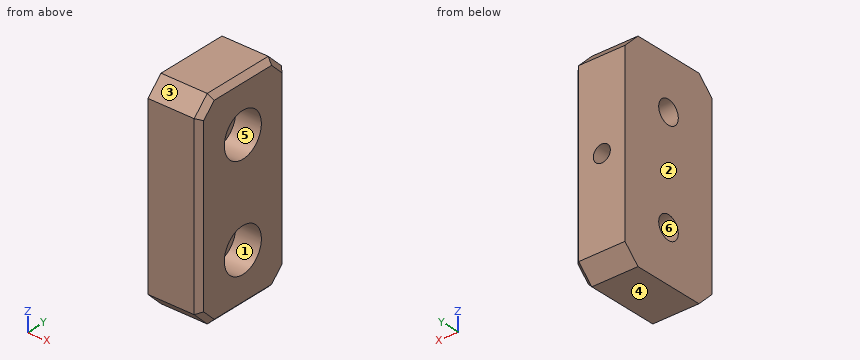
from build123d import *

# Parameters (mm, degrees)
SKETCH1_W           = 40
SKETCH1_H           = 20
BOSS_EXTRUDE1_DEPTH = 10
CHAMFER1_SIZE       = 3
CHAMFER2_SIZE       = 1
CUT_EXTRUDE1_DEPTH  = 10
CUT_EXTRUDE2_DEPTH  = 5
SKETCH3_R           = 1.65
CUT_EXTRUDE3_DEPTH  = 5


with BuildPart() as part:
    # Sketch1 → Boss-Extrude1 (new body)
    with BuildSketch(Plane(origin=(0, 0, 0), x_dir=(0, 0, -1), z_dir=(1, 0, 0))):
        Rectangle(SKETCH1_W, SKETCH1_H)
    extrude(amount=BOSS_EXTRUDE1_DEPTH)

    # Chamfer1
    chamfer1_edges = [part.edges().sort_by_distance(p)[0] for p in [
        (5, -10, -20),
        (5, -10, 20),
        (5, 10, 20),
        (5, 10, -20),
    ]]
    chamfer(chamfer1_edges, length=CHAMFER1_SIZE)

    # Chamfer2
    chamfer2_edges = [part.edges().sort_by_distance(p)[0] for p in [
        (10, 10, 0),
        (10, 0, -20),
        (10, 0, 20),
        (10, -10, 0),
        (10, 8.5, 18.5),
        (10, -8.5, 18.5),
        (10, -8.5, -18.5),
        (10, 8.5, -18.5),
    ]]
    chamfer(chamfer2_edges, length=CHAMFER2_SIZE)

    # Sketch2 → Cut-Extrude1 (cut)
    with BuildSketch(Plane(origin=(10, 0, 0), x_dir=(0, 0, -1), z_dir=(1, 0, 0))):
        with BuildLine():
            ThreePointArc((-12.25, 0), (-10, -2.25), (-7.75, 0))
            Line((-7.75, 0), (-12.25, 0))
        make_face()
        with BuildLine():
            Line((-12.25, 0), (-7.75, 0))
            ThreePointArc((-7.75, 0), (-10, 2.25), (-12.25, 0))
        make_face()
        with BuildLine():
            ThreePointArc((12.25, 0), (10, 2.25), (7.75, 0))
            Line((7.75, 0), (12.25, 0))
        make_face()
        with BuildLine():
            Line((12.25, 0), (7.75, 0))
            ThreePointArc((7.75, 0), (10, -2.25), (12.25, 0))
        make_face()
    extrude(amount=-CUT_EXTRUDE1_DEPTH, mode=Mode.SUBTRACT)

    # Sketch2_3 → Cut-Extrude2 (cut)
    with BuildSketch(Plane(origin=(10, 0, 0), x_dir=(0, 0, -1), z_dir=(1, 0, 0))):
        with BuildLine():
            ThreePointArc((-12.25, 0), (-10, 2.25), (-7.75, 0))
            Line((-7.75, 0), (-5.75, 0))
            ThreePointArc((-5.75, 0), (-10, 4.25), (-14.25, 0))
            Line((-14.25, 0), (-12.25, 0))
        make_face()
        with BuildLine():
            Line((-5.75, 0), (-7.75, 0))
            ThreePointArc((-7.75, 0), (-10, -2.25), (-12.25, 0))
            Line((-12.25, 0), (-14.25, 0))
            ThreePointArc((-14.25, 0), (-10, -4.25), (-5.75, 0))
        make_face()
        with BuildLine():
            ThreePointArc((14.25, 0), (10, 4.25), (5.75, 0))
            Line((5.75, 0), (7.75, 0))
            ThreePointArc((7.75, 0), (10, 2.25), (12.25, 0))
            Line((12.25, 0), (14.25, 0))
        make_face()
        with BuildLine():
            Line((7.75, 0), (5.75, 0))
            ThreePointArc((5.75, 0), (10, -4.25), (14.25, 0))
            Line((14.25, 0), (12.25, 0))
            ThreePointArc((12.25, 0), (10, -2.25), (7.75, 0))
        make_face()
    extrude(amount=-CUT_EXTRUDE2_DEPTH, mode=Mode.SUBTRACT)

    # Sketch3 → Cut-Extrude3 (cut)
    with BuildSketch(Plane(origin=(0, 10, 0), x_dir=(1, 0, 0), z_dir=(0, 1, 0))):
        with Locations((4.5, 0)):
            Circle(SKETCH3_R)
    extrude(amount=-CUT_EXTRUDE3_DEPTH, mode=Mode.SUBTRACT)


solid = part.part
The listing builds one solid part. Answer for the finished solid, in the listing's coordinates (mm). Face numbers are marked on the shaded views. A direction names the side the tool comes from. Give positions to 0.01 mm unless a question says otherwise; leave off trailing zeros. Loops run counter-clockwise (first coordinate to the right, second up) from the corner with the lowest first, then second, coordinate; pieces in that order, holes last. Notation, with made-up numbers: (-27, 44) - (30, 44) arc R10 ccw to (30, 48) - close; hole circle Ø2 at (70, 63.25). An arc over 180 degrees is marked (long way). Write each question's results on one line, items separated by ' | '.
1. Find section B-B, the plane y = -0.75. Write down the section's boundary in (x, z), then the cut area to 3 significant figures.
Resolved:
outline: (0, -20) - (9, -20) - (10, -19) - (10, -14.18) - (5, -14.18) - (5, -12.12) - (0, -12.12) - close; (0, -7.88) - (5, -7.88) - (5, -5.82) - (10, -5.82) - (10, 5.82) - (5, 5.82) - (5, 7.88) - (0, 7.88) - close; (0, 12.12) - (5, 12.12) - (5, 14.18) - (10, 14.18) - (10, 19) - (9, 20) - (0, 20) - close | area: 273 mm^2
2. Find section C-C, the plane x = 4.5. Write down the section's boundary in (y, z).
Resolved:
outline: (-10, -17) - (-7, -20) - (7, -20) - (10, -17) - (10, -1.65) - (5, -1.65) - (5, 1.65) - (10, 1.65) - (10, 17) - (7, 20) - (-7, 20) - (-10, 17) - close; hole circle Ø4.5 at (0, -10); hole circle Ø4.5 at (0, 10)
3. Which of the six approach directions +Z, -Z, +X, -X, +Y, -Y give full straight-line access (tool end or side, diameter ignored) to the marked faces 1 and 2?
Resolved:
face 1: +X | face 2: +Z, -Z, -X, +Y, -Y
4. Find section A-A, the plane z = 10. Write down the section's boundary in (x, y), then the cut area to 3 significant figures.
Resolved:
outline: (0, -10) - (9, -10) - (10, -9) - (10, -4.25) - (5, -4.25) - (5, -2.25) - (0, -2.25) - close; (0, 2.25) - (5, 2.25) - (5, 4.25) - (10, 4.25) - (10, 9) - (9, 10) - (0, 10) - close | area: 134 mm^2
5. Flat-ended cylindrical pins translate along their axes: P1, Ø1.6, axis at x = 4, z = 0, coming from the +Y side; P2, Ø3.5, axis at y = 0, z = -10, coming from the -X side; P3, Ø5, axis at y = 0, z = 10, coming from the +X side. Find the tip coordinate at first contact, or state that the pin passes through.
Resolved:
P1: stops at y = 5 | P2: passes through | P3: stops at x = 5
6. Consider probe 1 along Z at (x, y) = (7, 0); probe 2 along Z at (x, y) = (3, 0); probe 3 along Y at (x, z) = (6.25, 10). Determine where each line is inside the solid, lowest interval first. Write a range as from..to.
Resolved:
probe 1: z = -20..-14.25, -5.75..5.75, 14.25..20 | probe 2: z = -20..-12.25, -7.75..7.75, 12.25..20 | probe 3: y = -10..-4.25, 4.25..10
7. Find section D-D, the plane z = 0. Write down the section's boundary in (x, y).
Resolved:
outline: (0, -10) - (9, -10) - (10, -9) - (10, 9) - (9, 10) - (6.15, 10) - (6.15, 5) - (2.85, 5) - (2.85, 10) - (0, 10) - close
8. For a pull along Z with two mould halves and no side action, classify the marked faces 3, 4, 5 and 6 as +Z half, -Z half, draft (parallel to the pull), parting line (faces both ways), or undercut.
Resolved:
face 3: +Z half | face 4: -Z half | face 5: undercut | face 6: undercut
